Input: part model. Units: mm. Frame: model coordinates. A direction names the side the tool comes from. Coordinates: 2 decimals unless noted, no trailing zeros. Loops run counter-clockwise (first coordinate to the right, second up) from the corner with the lowest first, then second, coordinate; pieces in that order, holes last.
Item 1: Ray query, line 1 along Y through (x, z) = (-36, 1.45); line 2 along Y through (x, z) = (-31.75, 1.25); line 3 along X through (y, z) = (24.5, 0.9). Return the intervals inside material, ascending.
Item 2: Reachability of faces 1 (the flat face through (-35, -27.5, 1)), 2 (the flat face through (13, -30, 1)), 3 (the flat face through (25, 30, 1)) from +Z, -Z, +X, -X, +Y, -Y: full face, straight path, thin tool, end or side. Return the list, or none.
Item 3: Section C-C on x = -1. Return loops of the section in (y, z).
Item 4: Section D-D on y = 8.89. Return loops of the section in (x, z), and give its area (3 significant figures).
Item 5: Section A-A on y = 0. Return loops of the section in (x, z).
Item 6: Contact query for flat-ended pins moving along their axis: P1, Ø5, axis at x = -36, y = 23.5, coming from the -Z side; P2, Ø0.9, axis at y = -30, z = 2, coming from the +X side; P3, Ø1.5, axis at x = 36, z = 2, coming from the -Y side; P4, Ø1.5, axis at x = 33, z = 2.5, coming from the +Y side. Output: stop coordinate, or through.
Item 7: Pull-direction query (X, two-part tool) for faces 4 (the flat face through (46.5, 0, 1)), 5 (the cylindrical face through (-41.67, 24.81, 1.48)), 6 (the flat face through (19, -32.5, 1)); classes: released by +X, released by -X, zero draft, split by the parting line, or undercut.
Item 8: Section B-B on x = 36. Return loops of the section in (y, z), and give its area (3 significant figures).
```python
from build123d import *

# Parameters (mm, degrees)
ESQUISSE1_R        = 19
ESQUISSE1_R_2      = 1.55
BOSS_EXTRU_1_DEPTH = 3


with BuildPart() as part:
    # Esquisse1 → Boss.-Extru.1 (new body)
    with BuildSketch(Plane.XY):
        with BuildLine():
            Line((-25, -32.5), (-25, -27.5))
            Line((-25, -27.5), (-44.5, -27.5))
            ThreePointArc((-44.5, -27.5), (-45.914213562, -26.914213562), (-46.5, -25.5))
            Line((-46.5, -25.5), (-46.5, 25.5))
            ThreePointArc((-46.5, 25.5), (-45.914213562, 26.914213562), (-44.5, 27.5))
            Line((-44.5, 27.5), (-25, 27.5))
            Line((-25, 27.5), (-25, 32.5))
            Line((-25, 32.5), (-13, 32.5))
            Line((-13, 32.5), (-13, 27.5))
            Line((-13, 27.5), (13, 27.5))
            Line((13, 27.5), (13, 32.5))
            Line((13, 32.5), (25, 32.5))
            Line((25, 32.5), (25, 27.5))
            Line((25, 27.5), (44.5, 27.5))
            ThreePointArc((44.5, 27.5), (45.914213562, 26.914213562), (46.5, 25.5))
            Line((46.5, 25.5), (46.5, -25.5))
            ThreePointArc((46.5, -25.5), (45.914213562, -26.914213562), (44.5, -27.5))
            Line((44.5, -27.5), (25, -27.5))
            Line((25, -27.5), (25, -32.5))
            Line((25, -32.5), (13, -32.5))
            Line((13, -32.5), (13, -27.5))
            Line((13, -27.5), (-13, -27.5))
            Line((-13, -27.5), (-13, -32.5))
            Line((-13, -32.5), (-25, -32.5))
        make_face()
        Circle(ESQUISSE1_R, mode=Mode.SUBTRACT)
        with Locations((-42.5, 23.5)):
            Circle(ESQUISSE1_R_2, mode=Mode.SUBTRACT)
        with Locations((-36, 23.5)):
            Circle(ESQUISSE1_R_2, mode=Mode.SUBTRACT)
        with Locations((-31.75, 8.89)):
            Circle(ESQUISSE1_R_2, mode=Mode.SUBTRACT)
        with Locations((-31.75, -19.05)):
            Circle(ESQUISSE1_R_2, mode=Mode.SUBTRACT)
        with Locations((-36, -23.5)):
            Circle(ESQUISSE1_R_2, mode=Mode.SUBTRACT)
        with Locations((-42.5, -23.5)):
            Circle(ESQUISSE1_R_2, mode=Mode.SUBTRACT)
        with Locations((19.05, 24.13)):
            Circle(ESQUISSE1_R_2, mode=Mode.SUBTRACT)
        with Locations((36, 23.5)):
            Circle(ESQUISSE1_R_2, mode=Mode.SUBTRACT)
        with Locations((42.5, 23.5)):
            Circle(ESQUISSE1_R_2, mode=Mode.SUBTRACT)
        with Locations((42.5, -23.5)):
            Circle(ESQUISSE1_R_2, mode=Mode.SUBTRACT)
        with Locations((36, -23.5)):
            Circle(ESQUISSE1_R_2, mode=Mode.SUBTRACT)
        with Locations((20.32, -24.13)):
            Circle(ESQUISSE1_R_2, mode=Mode.SUBTRACT)
    extrude(amount=BOSS_EXTRU_1_DEPTH)


solid = part.part
```
Results found:
1. line 1: y = -27.5 to -25.05, -21.95 to 21.95, 25.05 to 27.5
1. line 2: y = -27.5 to -20.6, -17.5 to 7.34, 10.44 to 27.5
1. line 3: x = -46.5 to -43.68, -41.32 to -37.18, -34.82 to 17.54, 20.56 to 34.82, 37.18 to 41.32, 43.68 to 46.5
2. face 1: +Z, -Z, -X, -Y
2. face 2: +Z, -Z, -Y
2. face 3: +Z, -Z, +X, +Y
3. outline: (-27.5, 0) - (-18.97, 0) - (-18.97, 3) - (-27.5, 3) - close; (18.97, 0) - (27.5, 0) - (27.5, 3) - (18.97, 3) - close
4. outline: (-46.5, 0) - (-33.3, 0) - (-33.3, 3) - (-46.5, 3) - close; (-30.2, 0) - (-16.79, 0) - (-16.79, 3) - (-30.2, 3) - close; (16.79, 0) - (46.5, 0) - (46.5, 3) - (16.79, 3) - close
4. area: 169 mm2
5. outline: (-46.5, 0) - (-19, 0) - (-19, 3) - (-46.5, 3) - close; (19, 0) - (46.5, 0) - (46.5, 3) - (19, 3) - close
6. P1: stops at z = 0
6. P2: stops at x = 25
6. P3: stops at y = -27.5
6. P4: stops at y = 27.5
7. face 4: released by +X
7. face 5: undercut
7. face 6: zero draft
8. outline: (-27.5, 0) - (-25.05, 0) - (-25.05, 3) - (-27.5, 3) - close; (-21.95, 0) - (21.95, 0) - (21.95, 3) - (-21.95, 3) - close; (25.05, 0) - (27.5, 0) - (27.5, 3) - (25.05, 3) - close
8. area: 146 mm2
